from build123d import *

# Parameters (mm, degrees)
SKETCH1_W           = 127
SKETCH1_H           = 82.55
SKETCH1_R           = 6.985
BOSS_EXTRUDE1_DEPTH = 6.35
SKETCH2_W           = 31.75
SKETCH2_H           = 6.35
SKETCH2_W_2         = 25.4
BOSS_EXTRUDE2_DEPTH = 6.35
SKETCH3_W           = 27.94
SKETCH3_H           = 6.35
CUT_EXTRUDE1_DEPTH  = 6.35


with BuildPart() as part:
    # Sketch1 → Boss-Extrude1 (new body)
    with BuildSketch(Plane.XY):
        with Locations((-63.5, 41.275)):
            Rectangle(SKETCH1_W, SKETCH1_H)
        with Locations((-38.1, 41.275)):
            Circle(SKETCH1_R, mode=Mode.SUBTRACT)
        with Locations((-78.105, 41.275)):
            Circle(SKETCH1_R, mode=Mode.SUBTRACT)
    extrude(amount=BOSS_EXTRUDE1_DEPTH)

    # Sketch2 → Boss-Extrude2 (add)
    with BuildSketch(Plane(origin=(0, 0, 0), x_dir=(-1, 0, 0), z_dir=(0, 0, -1))):
        with Locations((15.875, -3.175)):
            Rectangle(SKETCH2_W, SKETCH2_H)
        with Locations((114.3, -3.175)):
            Rectangle(SKETCH2_W_2, SKETCH2_H)
    extrude(amount=-BOSS_EXTRUDE2_DEPTH)

    # Sketch3 → Cut-Extrude1 (cut)
    with BuildSketch(Plane(origin=(0, 0, 0), x_dir=(-1, 0, 0), z_dir=(0, 0, -1))):
        with Locations((26.67, 79.375)):
            Rectangle(SKETCH3_W, SKETCH3_H)
        with Locations((100.33, 79.375)):
            Rectangle(SKETCH3_W, SKETCH3_H)
    extrude(amount=-CUT_EXTRUDE1_DEPTH, mode=Mode.SUBTRACT)


solid = part.part
CAD build for the part. Positions are in the model's coordinates, mm. A direction names the side the tool comes from. Give positions to 0.01 mm unless a question says otherwise; leave off trailing zeros. Loops run counter-clockwise (first coordinate to the right, second up) from the corner with the lowest first, then second, coordinate; pieces in that order, holes last. Notation, with made-up numbers: M -14.75,13.25 L 4.25,13.25 A32 ccw 4.25,39.25 Z; hole C 47,30 d5. An arc over 180 degrees is marked long. One line per question, with ' | ' between items. Start each with the question number.
1. Saw through at D-D on x = -56.5. Give the cut face in (y, z).
2. 3-axis set-ups, long thin cutter, end or side, ignore diameter. For faces 1 (the face through (-67, 0, 3)), 2 (the face through (-6, 82.55, 3)), 3 (the face through (-26, 76.2, 3)): which of +Z, -Z, +X, -X, +Y, -Y reach the whole face in a straight line?
3. Saw through at C-C on x = -73. Give the cut face in (y, z).
4. Saw through at B-B on z = 3. Give the cut face in (x, y) (3 decimals), plus the area to 3 significant figures.
5. Saw through at A-A on x = -38.1. Give the cut face in (y, z), plus the area to 3 significant figures.
6. Probe L1, parallel to X at y = 77.5, z = 2.25; L2, parallel to X at y = 40, z = 2.75; L3, parallel to Y at x = -38.1, z = 3.75. List the from-to ranges inside material, lowest first. Write a range as from..to.
7. Flat gauge pins, fed straight in: pin 1 (3 mm diameter, centred on x = -32, z = 3.5, fed in from +Y); pin 2 (3 mm diameter, centred on x = -78, z = 3, fed in from -Y); pin 3 (11 mm diameter, centred on x = -78.105, y = 41.275, fed in from +Z). Where does each tip first touch, or does it go through?
8. Two-plate mould, pull along X, no slides. Class faces 4 (the face through (-12.7, 79, 3)), 5 (the face through (0, 37, 3)), 6 (the face through (-64, 82.55, 3)), 7 (the face through (-101.6, -3, 3)): pulls with the +X half, pulls with the -X half, needs draft (parallel to the pull), parting line crosses it, or undercut.
Result sheet:
1) outline: M 0,0 L 82.55,0 L 82.55,6.35 L 0,6.35 Z
2) face 1: +Z, -Z, -Y | face 2: +Z, -Z, +X, -X, +Y | face 3: +Z, -Z, +Y
3) outline: M 0,0 L 36.51,0 L 36.51,6.35 L 0,6.35 Z; M 46.04,0 L 82.55,0 L 82.55,6.35 L 46.04,6.35 Z
4) outline: M -127,-6.35 L -101.6,-6.35 L -101.6,0 L -31.75,0 L -31.75,-6.35 L 0,-6.35 L 0,82.55 L -12.7,82.55 L -12.7,76.2 L -40.64,76.2 L -40.64,82.55 L -86.36,82.55 L -86.36,76.2 L -114.3,76.2 L -114.3,82.55 L -127,82.55 Z; hole C -78.105,41.275 d13.97; hole C -38.1,41.275 d13.97 | area: 10,200 mm^2
5) outline: M 0,0 L 34.29,0 L 34.29,6.35 L 0,6.35 Z; M 48.26,0 L 76.2,0 L 76.2,6.35 L 48.26,6.35 Z | area: 395 mm^2
6) L1: x = -127..-114.3, -86.36..-40.64, -12.7..0 | L2: x = -127..-84.97, -71.24..-44.97, -31.23..0 | L3: y = 0..34.29, 48.26..76.2
7) pin 1: stops at y = 76.2 | pin 2: stops at y = 0 | pin 3: passes through
8) face 4: undercut | face 5: pulls with the +X half | face 6: needs draft | face 7: undercut
